Check sheet for the modelled part. Datum: model origin and axes. Units: mm. A direction names the side the tool comes from. Round coordinates to 2 decimals unless told otherwise and drop trailing zeros. Write each loop counter-clockwise with the first axis right and the second up, starting at its lowest first coordinate (ties: lowest second). Pieces come first, ordered by that corner, then holes. Notation, with made-up numbers: (-14.75, -40) -> (42.25, -40) arc R19 cw to (42.25, -29) -> close; hole circle Ø9 at (39.5, 88). An arc over 180 degrees is marked (long way). One line per item, written item: value.
from build123d import *

# Parameters (mm, degrees)
SKETCH1_R           = 2.5
BOSS_EXTRUDE1_DEPTH = 41
SKETCH2_R           = 3.5
BOSS_EXTRUDE2_DEPTH = 2
CHAMFER1_SIZE       = 1
SKETCH3_R           = 1.5
CUT_EXTRUDE1_DEPTH  = 5


with BuildPart() as part:
    # Sketch1 → Boss-Extrude1 (new body)
    with BuildSketch(Plane(origin=(0, 0, 0), x_dir=(1, 0, 0), z_dir=(0, 1, 0))):
        Circle(SKETCH1_R)
    extrude(amount=BOSS_EXTRUDE1_DEPTH)

    # Sketch2 → Boss-Extrude2 (add)
    with BuildSketch(Plane(origin=(0, 41, 0), x_dir=(1, 0, 0), z_dir=(0, 1, 0))):
        Circle(SKETCH2_R)
    extrude(amount=BOSS_EXTRUDE2_DEPTH)

    # Chamfer1
    chamfer1_edges = [part.edges().sort_by_distance(p)[0] for p in [
        (-3.5, 43, 0),
    ]]
    chamfer(chamfer1_edges, length=CHAMFER1_SIZE)

    # Sketch3 → Cut-Extrude1 (cut)
    with BuildSketch(Plane.XZ):
        Circle(SKETCH3_R)
    extrude(amount=-CUT_EXTRUDE1_DEPTH, mode=Mode.SUBTRACT)


solid = part.part
Item 1: Sectioned sample at B-B (x = 0). Enter the section's corners in (y, z).
Result set:
outline: (0, -2.5) -> (41, -2.5) -> (41, -3.5) -> (42, -3.5) -> (43, -2.5) -> (43, 2.5) -> (42, 3.5) -> (41, 3.5) -> (41, 2.5) -> (0, 2.5) -> (0, 1.5) -> (5, 1.5) -> (5, -1.5) -> (0, -1.5) -> close
Item 2: Tool access check on faces 1 (the flat face through (0, 5, 0)), 2 (the flat face through (0, 0, 2)). Record the directions out of +Z, -Z, +X, -X, +Y, -Y that give a thin tool (end or side, any length) a straight path to the whole face; none if there is none.
Result set:
face 1: -Y
face 2: +Z, -Z, +X, -X, -Y
Item 3: Depth check by flat-ended pin: pin 1 (2 mm diameter, centred on x = -2, y = 30.5, fed in from +Z); pin 2 (1.5 mm diameter, centred on x = -2, y = 21.5, fed in from +Z); pin 3 (0.9 mm diameter, centred on x = 0, z = 0, fed in from -Y). Enter the tip coordinate at first touch or a pass-through.
Result set:
pin 1: z = 2.29
pin 2: z = 2.17
pin 3: y = 5
Item 4: Sectioned sample at C-C (y = 32). Enter the section's corners in (x, z), then the cut area to 3 significant figures.
Result set:
outline: circle Ø5 at (0, 0)
area: 19.6 mm^2
Item 5: Release check for a two-part mould opening along X. For faces 3 (the cylindrical face through (3.233, 41.493, 1.341)), 4 (the flat face through (0, 43, 0)), 5 (the cylindrical face through (-1.5, 2.46, 0.07)) record: pulls with the +X half, pulls with the -X half, needs draft (parallel to the pull), parting line crosses it, or undercut.
Result set:
face 3: parting line crosses it
face 4: needs draft
face 5: undercut
Item 6: Material ranges on line 1 along Z through (x, y) = (0, 1.75); line 2 along X through (y, z) = (15.5, -2); line 3 along Z through (x, y) = (0, 11), recorded low to high.
Result set:
line 1: -2.5 to -1.5, 1.5 to 2.5
line 2: -1.5 to 1.5
line 3: -2.5 to 2.5
Item 7: Sectioned sample at A-A (z = 0). Enter the section's corners in (x, y).
Result set:
outline: (-3.5, 41) -> (-2.5, 41) -> (-2.5, 0) -> (-1.5, 0) -> (-1.5, 5) -> (1.5, 5) -> (1.5, 0) -> (2.5, 0) -> (2.5, 41) -> (3.5, 41) -> (3.5, 42) -> (2.5, 43) -> (-2.5, 43) -> (-3.5, 42) -> close
